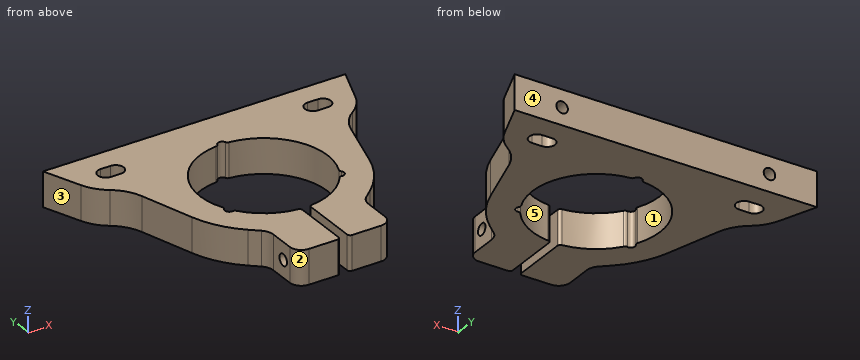
```python
from build123d import *

# Parameters (mm, degrees)
F1_DEPTH = 12
F2_R     = 5
F3_R     = 2
F4_DEPTH = 69.001
F5_R     = 4
F6_R     = 2
F7_DEPTH = 12
F8_R     = 1.5
F9_DEPTH = 25
F10_R    = 1


with BuildPart() as f1:
    # F0 (on Top) → F1 (new body)
    with BuildSketch(Plane.XY):
        with BuildLine():
            Line((52.5, 0), (-52.5, 0))
            Line((-52.5, 0), (-47.6682177495, -12.7529115916))
            ThreePointArc((-47.6682177495, -12.7529115916), (-45.4487126417, -16.689553935), (-42.1574376197, -19.7864660409))
            ThreePointArc((-42.1574376197, -19.7864660409), (-38.5340554499, -23.3236951077), (-36.2940938248, -27.8650010584))
            Line((-36.2940938248, -27.8650010584), (-30.8201520188, -46.3009960956))
            ThreePointArc((-30.8201520188, -46.3009960956), (-27.0602921577, -54.5098124511), (-21.1662026167, -61.3494703824))
            Line((-21.1662026167, -61.3494703824), (-16.5, -65.4307906954))
            Line((-16.5, -65.4307906954), (-16.5, -80.4307906954))
            Line((-16.5, -80.4307906954), (-1.5, -80.4307906954))
            Line((-1.5, -80.4307906954), (-1.5, -59.2491515674))
            ThreePointArc((-1.5, -59.2491515674), (0, -15), (1.5, -59.2491515674))
            Line((1.5, -59.2491515674), (1.5, -80.4307906954))
            Line((1.5, -80.4307906954), (16.5, -80.4307906954))
            Line((16.5, -80.4307906954), (16.5, -65.4307906954))
            Line((16.5, -65.4307906954), (21.1662026167, -61.3494703824))
            ThreePointArc((21.1662026167, -61.3494703824), (27.0602921577, -54.5098124511), (30.8201520188, -46.3009960956))
            Line((30.8201520188, -46.3009960956), (36.2940938248, -27.8650010584))
            ThreePointArc((36.2940938248, -27.8650010584), (38.5340554499, -23.3236951077), (42.1574376197, -19.7864660409))
            ThreePointArc((42.1574376197, -19.7864660409), (45.4487126417, -16.689553935), (47.6682177495, -12.7529115916))
            Line((47.6682177495, -12.7529115916), (52.5, 0))
        make_face()
        with BuildLine():
            Line((-34.2147789885, -13.5), (-37.6424851382, -13.5))
            ThreePointArc((-37.6424851382, -13.5), (-40.4638530749, -10.8213679366), (-37.7852210115, -8))
            Line((-37.7852210115, -8), (-34.2147789885, -8))
            ThreePointArc((-34.2147789885, -8), (-31.4647789885, -10.75), (-34.2147789885, -13.5))
        make_face(mode=Mode.SUBTRACT)
        with BuildLine():
            ThreePointArc((37.7852210115, -8), (40.4638530749, -10.8213679366), (37.6424851382, -13.5))
            Line((37.6424851382, -13.5), (34.2147789885, -13.5))
            ThreePointArc((34.2147789885, -13.5), (31.4647789885, -10.75), (34.2147789885, -8))
            Line((34.2147789885, -8), (37.7852210115, -8))
        make_face(mode=Mode.SUBTRACT)
    extrude(amount=F1_DEPTH)

    # F2
    f2_edges = [f1.edges().sort_by_distance(p)[0] for p in [
        (-16.5, -65.430791, 6),
        (16.5, -65.430791, 6),
    ]]
    fillet(f2_edges, radius=F2_R)

    # F3 (on face) → F4 (cut, through all)
    with BuildSketch(Plane(origin=(-16.5, 0, 0), x_dir=(0, -1, 0), z_dir=(-1, 0, 0))):
        with Locations((72.9307906954, 6)):
            Circle(F3_R)
    extrude(amount=-F4_DEPTH, mode=Mode.SUBTRACT)

    # F5
    f5_edges = [f1.edges().sort_by_distance(p)[0] for p in [
        (-16.5, -80.430791, 6),
        (16.5, -80.430791, 6),
    ]]
    fillet(f5_edges, radius=F5_R)

    # F6 (on face) → F7 (cut)
    with BuildSketch(Plane(origin=(0, 0, 0), x_dir=(-1, 0, 0), z_dir=(0, 1, 0))):
        with Locations((-36, 6)):
            Circle(F6_R)
        with Locations((36, 6)):
            Circle(F6_R)
    extrude(amount=-F7_DEPTH, mode=Mode.SUBTRACT)

    # F8 (on face) → F9 (cut)
    with BuildSketch(Plane.XY.offset(12)):
        with Locations((0, -15)):
            Circle(F8_R)
        with Locations((-19.1824626938, -48.225)):
            Circle(F8_R)
        with Locations((19.1824626938, -48.225)):
            Circle(F8_R)
    extrude(amount=-F9_DEPTH, mode=Mode.SUBTRACT)

    # F10
    f10_edges = [f1.edges().sort_by_distance(p)[0] for p in [
        (1.49914, -15.05079, 6),
        (-1.49914, -15.05079, 6),
        (-19.888047, -46.901312, 6),
        (-18.388907, -49.497898, 6),
        (18.388907, -49.497898, 6),
        (19.888047, -46.901312, 6),
        (1.5, -59.249152, 6),
        (-1.5, -59.249152, 6),
        (1.5, -80.430791, 6),
        (-1.5, -80.430791, 6),
    ]]
    fillet(f10_edges, radius=F10_R)


solid = f1.part
```
Here's how the part is built. I have some questions about the finished solid (model axes, mm). Face numbers are marked on the shaded views. A direction names the side the tool comes from. Coordinates: 2 decimals unless noted, no trailing zeros. Order: outer loops, then holes, each group sorted by start corner. A loop starts at its lowest first (then second) coordinate and runs counter-clockwise, first axis right, second up.
1) Imagine slicing it at C-C on y = -10.75. List the corners of the cut face in (x, z) for me, and give its area (3 significant figures).
2) Imagine slicing it at D-D on x = 6.5. List the corners of the cut face in (y, z) for me, and give its area (3 significant figures).
3) Which directions (+Z, -Z, +X, -X, +Y, -Y) give clear straight access to the entire face, cutting with the end or side of a thin tool? Please do the marked faces 1 and 2.
4) Will these pins go through, and if not, where does the flat tip stop? pin 1 (6 mm diameter, centred on y = -74, z = 5.5, fed in from +X); pin 2 (5 mm diameter, centred on x = 20.5, z = 5.5, fed in from -Y); pin 3 (2.5 mm diameter, centred on x = 35.5, z = 6, fed in from +Y).
5) Imagine slicing it at B-B on y = -40. List the corners of the cut face in (x, z) for me, and give its area (3 significant figures).
6) We'd pull the mould along X, two halves only. Please class the marked faces 3, 4 and 5: +X half, -X half, draft (parallel to the pull), parting line (faces both ways), or undercut.
7) Imagine slicing it at A-A on x = -15. List the corners of the cut face in (y, z) for me.
8) I need wall thicknesses on line 1 (X direction, y = -5, z = 5.5); line 2 (X direction, y = -73, z = 2.25); line 3 (X direction, y = -2.75, z = 6). Which ranges of each line are inside material? Lowest first, please.
Response values:
1. outline: (-48.43, 0) - (-40.46, 0) - (-40.46, 12) - (-48.43, 12) - close; (-31.46, 0) - (31.46, 0) - (31.46, 12) - (-31.46, 12) - close; (40.46, 0) - (48.43, 0) - (48.43, 12) - (40.46, 12) - close
1. area: 946 mm2
2. outline: (-80.43, 0) - (-58.32, 0) - (-58.32, 12) - (-80.43, 12) - close; (-15.98, 0) - (0, 0) - (0, 12) - (-15.98, 12) - close; hole circle Ø4 at (-72.93, 6)
2. area: 444 mm2
3. face 1: +Z, -Z
3. face 2: +Z, -Z, -X, -Y
4. pin 1: stops at x = 16.5
4. pin 2: stops at y = -64.13
4. pin 3: stops at y = -13.5
5. outline: (-32.69, 0) - (-21.97, 0) - (-21.97, 12) - (-32.69, 12) - close; (21.97, 0) - (32.69, 0) - (32.69, 12) - (21.97, 12) - close
5. area: 257 mm2
6. face 3: -X half
6. face 4: draft
6. face 5: undercut
7. outline: (-79.55, 0) - (-53.45, 0) - (-53.45, 12) - (-79.55, 12) - close; (-20.85, 0) - (0, 0) - (0, 12) - (-20.85, 12) - close; hole circle Ø4 at (-72.93, 6)
8. line 1: x = -50.61 to -37.94, -34.06 to 34.06, 37.94 to 50.61
8. line 2: x = -16.5 to -1.5, 1.5 to 16.5
8. line 3: x = -51.46 to -38, -34 to 34, 38 to 51.46
